```python
from build123d import *

# Parameters (mm, degrees)
ESQUISSE1_R             = 17.45
ESQUISSE1_R_2           = 15.45
BOSS_EXTRU_1_DEPTH      = 50
ENL_V_MAT_EXTRU_1_REACH = 41.698
ENL_V_MAT_EXTRU_2_REACH = 39.706
ENL_V_MAT_EXTRU_3_REACH = 43.998


with BuildPart() as part:
    # Esquisse1 → Boss.-Extru.1 (new body)
    with BuildSketch(Plane.XY):
        Circle(ESQUISSE1_R)
        Circle(ESQUISSE1_R_2, mode=Mode.SUBTRACT)
    extrude(amount=-BOSS_EXTRU_1_DEPTH)

    # Esquisse2 → Enl_v. mat.-Extru.1 (cut, up to next)
    with BuildSketch(Plane(origin=(-5.845108935, -16.388859068, 0), x_dir=(-0.941888452, 0.335925801, 0), z_dir=(-0.335925801, -0.941888452, 0)), mode=Mode.PRIVATE) as enl_v_mat_extru_1_sk1:
        with BuildLine():
            Line((1.7, 28.5), (1.7, 21.5))
            ThreePointArc((1.7, 21.5), (0, 19.8), (-1.7, 21.5))
            Line((-1.7, 21.5), (-1.7, 28.5))
            ThreePointArc((-1.7, 28.5), (0, 30.2), (1.7, 28.5))
        make_face()
    enl_v_mat_extru_1_tool1 = extrude(enl_v_mat_extru_1_sk1.sketch, amount=-ENL_V_MAT_EXTRU_1_REACH, mode=Mode.PRIVATE) & part.part
    add(enl_v_mat_extru_1_tool1.solids().sort_by_distance((-5.845109, -16.388859, -25))[0], mode=Mode.SUBTRACT)

    # Esquisse4 → Enl_v. mat.-Extru.2 (cut, up to next)
    with BuildSketch(Plane(origin=(17.115722759, 3.132416708, 0), x_dir=(0, 0, 1), z_dir=(0.983662228, 0.180023949, 0)), mode=Mode.PRIVATE) as enl_v_mat_extru_2_sk1:
        with BuildLine():
            Line((-28.5, 1.71), (-21.5, 1.71))
            ThreePointArc((-21.5, 1.71), (-19.79, 0), (-21.5, -1.71))
            Line((-21.5, -1.71), (-28.5, -1.71))
            ThreePointArc((-28.5, -1.71), (-30.21, 0), (-28.5, 1.71))
        make_face()
    enl_v_mat_extru_2_tool1 = extrude(enl_v_mat_extru_2_sk1.sketch, amount=-ENL_V_MAT_EXTRU_2_REACH, mode=Mode.PRIVATE) & part.part
    add(enl_v_mat_extru_2_tool1.solids().sort_by_distance((17.115723, 3.132417, -25))[0], mode=Mode.SUBTRACT)

    # Esquisse5 → Enl_v. mat.-Extru.3 (cut, up to next)
    with BuildSketch(Plane(origin=(-11.270613824, 13.256442359, 0), x_dir=(0, 0, 1), z_dir=(-0.647736427, 0.761864503, 0)), mode=Mode.PRIVATE) as enl_v_mat_extru_3_sk1:
        with BuildLine():
            Line((-28.5, 1.72), (-21.5, 1.72))
            ThreePointArc((-21.5, 1.72), (-19.78, 0), (-21.5, -1.72))
            Line((-21.5, -1.72), (-28.5, -1.72))
            ThreePointArc((-28.5, -1.72), (-30.22, 0), (-28.5, 1.72))
        make_face()
    enl_v_mat_extru_3_tool1 = extrude(enl_v_mat_extru_3_sk1.sketch, amount=-ENL_V_MAT_EXTRU_3_REACH, mode=Mode.PRIVATE) & part.part
    add(enl_v_mat_extru_3_tool1.solids().sort_by_distance((-11.270614, 13.256442, -25))[0], mode=Mode.SUBTRACT)


solid = part.part
```
CAD build for the part. Positions are in the model's coordinates, mm. A direction names the side the tool comes from. Round coordinates to 2 decimals unless told otherwise and drop trailing zeros. Order: outer loops, then holes, each group sorted by start corner. A loop starts at its lowest first (then second) coordinate and runs counter-clockwise, first axis right, second up. Notation, with made-up numbers: (77.25, 42.25) -> (101.25, 42.25) arc R22 ccw to (101.25, 49.25) -> close; hole circle Ø9 at (85.5, -20.75). An arc over 180 degrees is marked (long way). One line per question, with ' | ' between items.
Q1. Drop flat-ended pins along their axis: pin 1 (8 mm diameter, centred on x = -14, z = -29, fed in from +Y); pin 2 (10 mm diameter, centred on y = 11.5, z = -41, fed in from +X); pin 3 (12 mm diameter, centred on x = -4, y = -9, fed in from -Z); pin 4 (1 mm diameter, centred on x = -12.5, z = -27, fed in from +Y). Give the stop position or say it passes through.
Completed:
pin 1: stops at y = 14.3 | pin 2: stops at x = 16.19 | pin 3: stops at z = -50 | pin 4: stops at y = 12.67
Q2. Probe probe 1 along Y at (x, z) = (0, -27); probe 2 along Y at (x, z) = (-14, -13.5); probe 3 along X at (y, z) = (-1, -33.5). List the from-to ranges inside material, lowest first.
Completed:
probe 1: y = -17.45 to -15.45, 15.45 to 17.45 | probe 2: y = -10.42 to -6.53, 6.53 to 10.42 | probe 3: x = -17.42 to -15.42, 15.42 to 17.42
Q3. Slice it at A-A (y = 0). Write the cut outline in (x, z), then the cut area to 3 significant figures.
Completed:
outline: (-17.45, -50) -> (-15.45, -50) -> (-15.45, 0) -> (-17.45, 0) -> close; (15.45, -50) -> (17.45, -50) -> (17.45, 0) -> (15.45, 0) -> close | area: 200 mm^2
Q4. Slice it at C-C (z = -7). Write the cut outline in (x, y).
Completed:
outline: circle Ø34.9 at (0, 0); hole circle Ø30.9 at (0, 0)
Q5. Which spindle directions (+Z, -Z, +X, -X, +Y, -Y) get a long thin tool onto all of the face, cutting with end or side? Do faces 4 (the cylindrical face through (-12.26, -9.4, -24.65)), 5 (the cylindrical face through (16.13, 2.91, -19.79)). Say none if no direction does.
Completed:
face 4: +Z, -Z | face 5: none
Q6. Two-plate mould, pull along X, no slides. Class faces 1 (the cylindrical face through (-3.783, -17.035, -24.65)), 2 (the flat face through (-10, -12, -50)), 3 (the cylindrical face through (-10.65, 12.46, -30.22)): released by +X, released by -X, zero draft, split by the parting line, or undercut.
Completed:
face 1: split by the parting line | face 2: zero draft | face 3: undercut
